Part model, mm, in its own coordinate system. Coordinates: 2 decimals unless noted, no trailing zeros. Order: outer loops, then holes, each group sorted by start corner. A loop starts at its lowest first (then second) coordinate and runs counter-clockwise, first axis right, second up. Notation, with made-up numbers: (52, 42.5) - (67, 42.5) arc R28 ccw to (67, 66.5) - close; hole circle Ø2 at (-10, 5.5). An arc over 180 degrees is marked (long way). Use a Markdown table: item, result. Add a question column.
1) Wall check: L1, parallel to X at y = 65, z = 7.25; L2, parallel to Z at x = 0.3, y = 66.75. Give the ranges that are in metal, low to high. Write a range as [from, to].
2) Saw through at A-A on y = 10.5. List the corners of the cut face in (x, z).
3) Drop flat-ended pins along their axis: P1, Ø4, axis at x = 4.5, y = 69, coming from the +Z side; P2, Ø4.5, axis at y = 6.75, z = 4.5, coming from the -X side. Give the stop position or say it passes through.
4) Saw through at B-B on z = 4.5. Count the separate pieces of the cut face and the enclosed holes in it, then the cut area to 3 significant figures.
Autodesk Inventor part; units mm, degrees
ref_plane "YZ Plane" through (0, 0, 0) normal (1, 0, 0) x (0, 1, 0)
ref_plane "XZ Plane" through (0, 0, 0) normal (0, 1, 0) x (-1, 0, 0)
ref_plane "XY Plane" through (0, 0, 0) normal (0, 0, 1) x (1, 0, 0)
sketch "スケッチ1" plane through (0, 0, 0) normal (0, 1, 0) x (-1, 0, 0)
  line L0 (0, 0) -> (-9, 0)
  line L1 (-9, 0) -> (-9, 9)
  line L2 (-9, 9) -> (0, 9)
  line L3 (0, 9) -> (0, 0)
  line L4 (-1.2, 7.8) -> (-7.8, 7.8)
  line L5 (-7.8, 7.8) -> (-7.8, 1.2)
  line L6 (-7.8, 1.2) -> (-1.2, 1.2)
  line L7 (-1.2, 1.2) -> (-1.2, 7.8)
  dimension "d0" = 9
  dimension "d1" = 9
  dimension "d2" = 1.2
  dimension "d3" = 1.2
  dimension "d4" = 1.2
  dimension "d5" = 1.2
extrude "押し出し1" add sketch "スケッチ1" along normal blind 73.5
sketch "スケッチ2" plane through (0, 0, 9) normal (0, 0, 1) x (1, 0, 0)
  line L0 (0, 0) -> (0, 73.5)
  line L1 (0, 0) -> (9, 0)
  line L2 (0, 73.5) -> (9, 73.5)
  point P0 (4.5, 69)
  point P1 (4.5, 4.5)
  dimension "d8" = 4.5
  dimension "d9" = 4.5
  dimension "d10" = 4.5
  dimension "d11" = 4.5
hole "穴1" at (4.5, 69, 9) at (4.5, 4.5, 9) direction (0, 0, -1) diameter 3.3 end through all
sketch "スケッチ3" plane through (9, 0, 9) normal (1, 0, 0) x (0, 0, -1)
  line L0 (0, 0) -> (0, 73.5)
  line L1 (0, 73.5) -> (9, 73.5)
  line L2 (0, 0) -> (9, 0)
  point P0 (4.5, 60)
  point P1 (4.5, 13.5)
  dimension "d19" = 4.5
  dimension "d20" = 4.5
  dimension "d21" = 13.5
  dimension "d22" = 13.5
hole "穴2" at (9, 60, 4.5) at (9, 13.5, 4.5) direction (-1, 0, 0) diameter 3.3 end through all
sketch "スケッチ4" plane through (9, 0, 0) normal (0, 0, -1) x (-1, 0, 0)
  line L0 (9, 0) -> (9, 73.5)
  line L1 (0, 73.5) -> (9, 73.5)
  line L2 (0, 0) -> (9, 0)
  point P0 (4.5, 48.5)
  point P1 (4.5, 25)
  dimension "d30" = 4.5
  dimension "d31" = 4.5
  dimension "d32" = 25
  dimension "d33" = 25
hole "穴3" at (4.5, 48.5, 0) at (4.5, 25, 0) direction (0, 0, 1) diameter 4 end through all
sketch "スケッチ5" plane through (0, 0, 9) normal (0, 0, 1) x (1, 0, 0)
  circle A0 centre (4.5, 25) radius 2
  circle A1 centre (4.5, 4.5) radius 1.65
  circle A2 centre (4.5, 48.5) radius 2
  line L0 (0, 0) -> (0, 73.5)
  point P0 (4.5, 11.3333)
  point P1 (4.5, 18.1667)
  point P2 (4.5, 32.8333)
  point P3 (4.5, 55.3333)
  point P4 (4.5, 62.1667)
  point P5 (4.5, 40.6667)
  dimension "d41" = 20.5
  dimension "d42" = 23.5
  dimension "d43" = 4.5
  dimension "d44" = 4.5
  dimension "d45" = 6.8333
  dimension "d46" = 6.8333
  dimension "d47" = 4.5
  dimension "d48" = 7.8333
  dimension "d49" = 7.8333
  dimension "d50" = 6.8333
  dimension "d51" = 6.8333
  dimension "d52" = 4.5
  dimension "d53" = 4.5
  dimension "d54" = 4.5
hole "穴4" at (4.5, 11.3333, 9) at (4.5, 18.1667, 9) at (4.5, 32.8333, 9) at (4.5, 55.3333, 9) at (4.5, 62.1667, 9) at (4.5, 40.6667, 9) direction (0, 0, -1) diameter 5 end through all
sketch "スケッチ6" plane through (0, 0, 0) normal (-1, 0, 0) x (0, 0, 1)
  line L0 (9, 0) -> (9, 73.5)
  circle A0 centre (4.5, 13.5) radius 1.65
  line L1 (0, 0) -> (9, 0)
  circle A1 centre (4.5, 60) radius 1.65
  point P0 (4.5, 66.75)
  point P1 (4.5, 6.75)
  dimension "d62" = 4.5
  dimension "d63" = 4.5
  dimension "d64" = 13.5
  dimension "d65" = 6.75
  dimension "d66" = 6.75
hole "穴5" at (0, 66.75, 4.5) at (0, 6.75, 4.5) direction (1, 0, 0) diameter 5 end through all
sketch "スケッチ7" plane through (0, 0, 0) normal (-1, 0, 0) x (0, 0, 1)
  line L0 (9, 0) -> (9, 73.5)
  circle A0 centre (4.5, 60) radius 1.65
  point P0 (0, 0)
  point P1 (4.5, 54.9649)
  point P2 (4.5, 49.9649)
  point P3 (4.5, 44.9649)
  point P4 (4.5, 39.9649)
  point P5 (4.5, 34.9649)
  point P6 (4.5, 29.9649)
  point P7 (4.5, 24.9649)
  point P8 (4.5, 19.9649)
  dimension "d74" = 4.5
  dimension "d75" = 5.0351
  dimension "d78" = 5
hole "穴6" at (0, 54.9649, 4.5) at (0, 49.9649, 4.5) at (0, 44.9649, 4.5) at (0, 39.9649, 4.5) at (0, 34.9649, 4.5) at (0, 29.9649, 4.5) at (0, 24.9649, 4.5) at (0, 19.9649, 4.5) direction (1, 0, 0) diameter 4 end through all
equation "\"d3\" = d2"
equation "\"d4\" = d3"
equation "\"d5\" = d4"
properties part number "ハンド9x9_3" material "アルミニウム 6061"
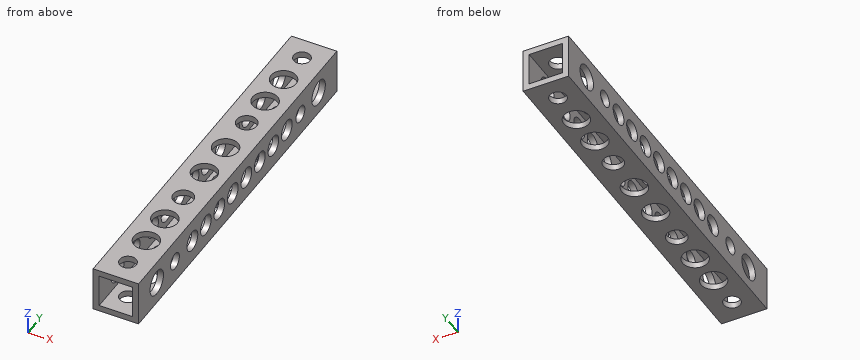
Results are:
| question | item | result |
|---|---|---|
| 1 | L1 | [0, 1.2], [7.8, 9] |
| 1 | L2 | [0, 2], [7, 9] |
| 2 | outline | (0, 0) - (2.14, 0) - (2.14, 1.2) - (1.2, 1.2) - (1.2, 7.8) - (2.14, 7.8) - (2.14, 9) - (0, 9) - close; (6.86, 0) - (9, 0) - (9, 9) - (6.86, 9) - (6.86, 7.8) - (7.8, 7.8) - (7.8, 1.2) - (6.86, 1.2) - close |
| 3 | P1 | z = 9 |
| 3 | P2 | through |
| 4 | separate pieces | 26 |
| 4 | enclosed holes | 0 |
| 4 | area | 59.8 mm2 |
